Source: CAD feature listing. Evaluate the final solid. Frame: model axes, mm. A direction names the side the tool comes from. Give positions to 0.01 mm unless a question says otherwise; leave off trailing zeros. Order: outer loops, then holes, each group sorted by start corner. A loop starts at its lowest first (then second) coordinate and runs counter-clockwise, first axis right, second up. Notation, with made-up numbers: M -10.5,84.5 L -0.5,84.5 A14 cw -0.5,97.5 Z; hole C -25,-33 d11. An arc over 180 degrees is marked long. Answer as a JSON object with one key per item and string values. Group by question number.
1. Material intervals for L1, parallel to X at y = -41.5, z = 0; L2, parallel to X at y = 12.5, z = 1.5; L3, parallel to X at y = -34, z = 3, sorted ascending. Write a range as [from, to].
2. Section query A-A (y = 4). Output: boundary loops of the cut face in (x, z), plus the area to 3 significant figures.
3. Section query B-B (z = 4). Count the separate pieces of the cut face and the enclosed holes in it, plus the area to 3 significant figures.
4. Set-up query: faces 1 (the flat face through (-24.5, -39.26, 0.18)), 2 (the cylindrical face through (-16.26, 39.482, 0.175)), 3 (the cylindrical face through (-36.09, -13.83, -0.18)), 4 (the flat face through (-39.26, 24.5, 0.18)). Return all of +Z, -Z, +X, -X, +Y, -Y with unobstructed straight access to the full face (end or side cutting, diameter ignored); none if empty.
5. Pin query (flat end, axial travel): P1, Ø1.5, axis at y = 3, z = 3.5, coming from the +X side; P2, Ø5, axis at x = -33, z = 2, coming from the +Y side; P3, Ø5, axis at y = 25, z = 8, coming from the +X side. Return the tip coordinate at first contact, or that it passes through.
6. Pull-direction query (Y, two-part tool) for faces 5 (the flat face through (22, -10, 12.5)), 6 (the cylindrical face through (-25.35, -10.38, -0.18)), 7 (the flat face through (31.253, 38.531, 0.175)); classes: +Y half, -Y half, draft (parallel to the pull), parting line (faces both ways), or undercut.
from build123d import *

# Parameters (mm, degrees)
F1_R     = 2.1084229829
F1_R_2   = 2.1529922124
F1_R_3   = 6.765859494
F1_R_4   = 23.4458713357
F2_DEPTH = 12.5


# Not quite as in the source:
# - ends of sketch curves that miss each other by under 0.0002 mm in the source are joined


with BuildPart() as f2:
    # F1 (on Top) → F2 (new body, symmetric)
    with BuildSketch(Plane.XY):
        with BuildLine():
            Line((10.4387272149, 48.6714951694), (-2.1118e-06, 50))
            Line((-2.1118e-06, 50), (-10.4387272149, 48.6714951694))
            Line((-10.4387272149, 48.6714951694), (-10.4387272149, 41.4038337767))
            ThreePointArc((-10.4387272149, 41.4038337767), (-16.3403785702, 39.4491635584), (-21.89563683, 36.6582264313))
            Line((-21.89563683, 36.6582264313), (-27.0346494841, 41.7972390854))
            Line((-27.0346494841, 41.7972390854), (-35.3553405526, 35.355337566))
            Line((-35.3553405526, 35.355337566), (-41.7972390854, 27.0346494841))
            Line((-41.7972390854, 27.0346494841), (-36.6582264313, 21.89563683))
            ThreePointArc((-36.6582264313, 21.89563683), (-39.4491635584, 16.3403785702), (-41.4038337767, 10.4387272149))
            Line((-41.4038337767, 10.4387272149), (-48.6714951694, 10.4387272149))
            Line((-48.6714951694, 10.4387272149), (-50, -2.1118e-06))
            Line((-50, -2.1118e-06), (-48.6714951694, -10.4387272149))
            Line((-48.6714951694, -10.4387272149), (-41.4038337767, -10.4387272149))
            ThreePointArc((-41.4038337767, -10.4387272149), (-39.4491635584, -16.3403785702), (-36.6582264313, -21.89563683))
            Line((-36.6582264313, -21.89563683), (-41.7972390854, -27.0346494841))
            Line((-41.7972390854, -27.0346494841), (-35.355337566, -35.3553405526))
            Line((-35.355337566, -35.3553405526), (-27.0346494841, -41.7972390854))
            Line((-27.0346494841, -41.7972390854), (-21.89563683, -36.6582264313))
            ThreePointArc((-21.89563683, -36.6582264313), (-16.3403785702, -39.4491635584), (-10.4387272149, -41.4038337767))
            Line((-10.4387272149, -41.4038337767), (-10.4387272149, -48.6714951694))
            Line((-10.4387272149, -48.6714951694), (2.1118e-06, -50))
            Line((2.1118e-06, -50), (10.4387272149, -48.6714951694))
            Line((10.4387272149, -48.6714951694), (10.4387272149, -41.4038337767))
            ThreePointArc((10.4387272149, -41.4038337767), (16.3403785702, -39.4491635584), (21.89563683, -36.6582264313))
            Line((21.89563683, -36.6582264313), (27.0346494841, -41.7972390854))
            Line((27.0346494841, -41.7972390854), (35.3553405526, -35.355337566))
            Line((35.3553405526, -35.355337566), (41.7972390854, -27.0346494841))
            Line((41.7972390854, -27.0346494841), (36.6582264313, -21.89563683))
            ThreePointArc((36.6582264313, -21.89563683), (39.4491635584, -16.3403785702), (41.4038337767, -10.4387272149))
            Line((41.4038337767, -10.4387272149), (48.6714951694, -10.4387272149))
            Line((48.6714951694, -10.4387272149), (50, 2.1118e-06))
            Line((50, 2.1118e-06), (48.6714951694, 10.4387272149))
            Line((48.6714951694, 10.4387272149), (41.4038337767, 10.4387272149))
            ThreePointArc((41.4038337767, 10.4387272149), (39.4491635584, 16.3403785702), (36.6582264313, 21.89563683))
            Line((36.6582264313, 21.89563683), (41.7972390854, 27.0346494841))
            Line((41.7972390854, 27.0346494841), (35.355337566, 35.3553405526))
            Line((35.355337566, 35.3553405526), (27.0346494841, 41.7972390854))
            Line((27.0346494841, 41.7972390854), (21.89563683, 36.6582264313))
            ThreePointArc((21.89563683, 36.6582264313), (16.3403785702, 39.4491635584), (10.4387272149, 41.4038337767))
            Line((10.4387272149, 41.4038337767), (10.4387272149, 48.6714951694))
        make_face()
        with Locations((-14.1885686223, -33.8735479302)):
            Circle(F1_R, mode=Mode.SUBTRACT)
        with Locations((-11.5808588113, -27.1737373769)):
            Circle(F1_R_2, mode=Mode.SUBTRACT)
        with Locations((-33.9850485325, -13.9193823561)):
            Circle(F1_R, mode=Mode.SUBTRACT)
        with Locations((-27.4036377668, -11.025830172)):
            Circle(F1_R_2, mode=Mode.SUBTRACT)
        with Locations((-23.7041544531, -23.7041544531)):
            Circle(F1_R_3, mode=Mode.SUBTRACT)
        with Locations((0, -33.5227367122)):
            Circle(F1_R_3, mode=Mode.SUBTRACT)
        with Locations((11.025830172, -27.4036377668)):
            Circle(F1_R_2, mode=Mode.SUBTRACT)
        with Locations((13.9193823561, -33.9850485325)):
            Circle(F1_R, mode=Mode.SUBTRACT)
        with Locations((23.7041544531, -23.7041544531)):
            Circle(F1_R_3, mode=Mode.SUBTRACT)
        with Locations((33.8735479302, -14.1885686223)):
            Circle(F1_R, mode=Mode.SUBTRACT)
        with Locations((27.1737373769, -11.5808588113)):
            Circle(F1_R_2, mode=Mode.SUBTRACT)
        with Locations((-33.5227367122, 0)):
            Circle(F1_R_3, mode=Mode.SUBTRACT)
        with Locations((-27.1737373769, 11.5808588113)):
            Circle(F1_R_2, mode=Mode.SUBTRACT)
        with Locations((-33.8735479302, 14.1885686223)):
            Circle(F1_R, mode=Mode.SUBTRACT)
        with Locations((-23.7041544531, 23.7041544531)):
            Circle(F1_R_3, mode=Mode.SUBTRACT)
        with Locations((-13.9193823561, 33.9850485325)):
            Circle(F1_R, mode=Mode.SUBTRACT)
        with Locations((-11.025830172, 27.4036377668)):
            Circle(F1_R_2, mode=Mode.SUBTRACT)
        Circle(F1_R_4, mode=Mode.SUBTRACT)
        with Locations((23.7041544531, 23.7041544531)):
            Circle(F1_R_3, mode=Mode.SUBTRACT)
        with Locations((33.5227367122, 0)):
            Circle(F1_R_3, mode=Mode.SUBTRACT)
        with Locations((27.4036377668, 11.025830172)):
            Circle(F1_R_2, mode=Mode.SUBTRACT)
        with Locations((33.9850485325, 13.9193823561)):
            Circle(F1_R, mode=Mode.SUBTRACT)
        with Locations((11.5808588113, 27.1737373769)):
            Circle(F1_R_2, mode=Mode.SUBTRACT)
        with Locations((0, 33.5227367122)):
            Circle(F1_R_3, mode=Mode.SUBTRACT)
        with Locations((14.1885686223, 33.8735479302)):
            Circle(F1_R, mode=Mode.SUBTRACT)
    extrude(amount=F2_DEPTH, both=True)


solid = f2.part
Answer sheet:
{
 "1": {"L1": "[-27.42, -26.74], [-10.44, 10.44], [26.74, 27.42]", "L2": "[-40.83, -35.14], [-32.61, -29.12], [-25.23, -19.84], [19.84, 25.83], [28.97, 32.43], [35.54, 40.83]", "L3": "[-36.4, -16.29], [-12.08, -6.75], [6.75, 11.81], [16.03, 36.4]"},
 "2": {"outline": "M -49.49,-12.5 L -38.98,-12.5 L -38.98,12.5 L -49.49,12.5 Z; M -28.07,-12.5 L -23.1,-12.5 L -23.1,12.5 L -28.07,12.5 Z; M 23.1,-12.5 L 28.07,-12.5 L 28.07,12.5 L 23.1,12.5 Z; M 38.98,-12.5 L 49.49,-12.5 L 49.49,12.5 L 38.98,12.5 Z", "area": "774 mm^2"},
 "3": {"separate pieces": "1", "enclosed holes": "25", "area": "3,800 mm^2"},
 "4": {"face 1": "+Z, -Z, -Y", "face 2": "+Z, -Z, +Y", "face 3": "+Z, -Z", "face 4": "+Z, -Z, -X"},
 "5": {"P1": "x = 49.71", "P2": "y = 39.11", "P3": "x = 41.8"},
 "6": {"face 5": "draft", "face 6": "undercut", "face 7": "+Y half"}
}
